Can you work these out from the drawing? Everything is in mm from the part's minimum corner. Give positions to 0.01 mm unless a question says otherwise; leave off trailing zeros. Order: outer loops, then holes, each group sorted by start corner. A loop starts at its lowest first (then second) coordinate and runs counter-clockwise, first axis right, second up. Notation, with made-up numbers: M 80.25,0 L 87.25,0 A22 ccw 87.25,8 Z; hole C 70,30 d6. An arc over 180 degrees is marked long. Use a Markdown table: item, result. Add a question column.
Item 1: I'm going to push flat-ended pins straight in: pin 1 Ø1 at (y, z) = (44, 2) entering from -X; pin 2 Ø0.9 at (x, z) = (38.5, 1.5) entering from +Y; pin 3 Ø1 at (y, z) = (2, 1) entering from +X. Where does each tip first touch, or does it pass through?
Item 2: Suppose I cut it at B-B on x = 29.5. Write out the boundary of the cut face in (y, z), plus the area to 3 significant figures.
Item 3: Suppose I cut it at C-C on z = 1.5. Count the separate pieces of the cut face and the enclosed holes in it, plus the area to 3 significant figures.
Item 4: Suppose I cut it at A-A on y = 31. Write out the boundary of the cut face in (x, z).
Item 5: If I drill on L1, parallel to Y at x = 57, z = 1.65; L2, parallel to X at y = 26, z = 2.1; L3, parallel to Y at x = 17, z = 1.45, over which ranges is the centre line in solid material (lowest first)? Write a range as from..to.
Item 6: Suppose I cut it at D-D on x = 7.5. Write out the boundary of the cut face in (y, z) (3 decimals).
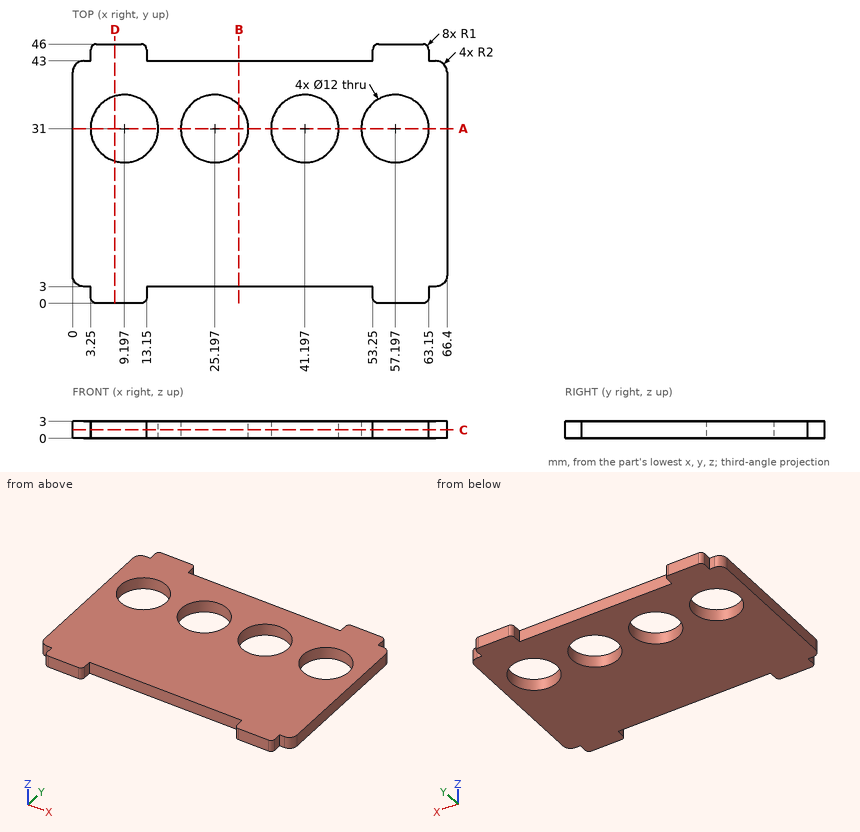
Findings below:
| question | item | result |
|---|---|---|
| 1 | pin 1 | stops at x = 3.25 |
| 1 | pin 2 | stops at y = 43 |
| 1 | pin 3 | stops at x = 63.15 |
| 2 | outline | M 3,0 L 26.82,0 L 26.82,3 L 3,3 Z; M 35.18,0 L 43,0 L 43,3 L 35.18,3 Z |
| 2 | area | 94.9 mm^2 |
| 3 | separate pieces | 1 |
| 3 | enclosed holes | 4 |
| 3 | area | 2,320 mm^2 |
| 4 | outline | M 0,0 L 3.2,0 L 3.2,3 L 0,3 Z; M 15.2,0 L 19.2,0 L 19.2,3 L 15.2,3 Z; M 31.2,0 L 35.2,0 L 35.2,3 L 31.2,3 Z; M 47.2,0 L 51.2,0 L 51.2,3 L 47.2,3 Z; M 63.2,0 L 66.4,0 L 66.4,3 L 63.2,3 Z |
| 5 | L1 | y = 0..25, 37..46 |
| 5 | L2 | x = 0..5.88, 12.51..21.88, 28.51..37.88, 44.51..53.88, 60.51..66.4 |
| 5 | L3 | y = 3..43 |
| 6 | outline | M 0,0 L 25.245,0 L 25.245,3 L 0,3 Z; M 36.755,0 L 46,0 L 46,3 L 36.755,3 Z |
